```python
from build123d import *

# Parameters (mm, degrees)
F1_DEPTH = 127
F1_TAPER = -10
F2_R     = 7.8205252783
F3_DEPTH = 127.0010001
F4_R     = 16.8280941537
F5_DEPTH = 127.0010001
F6_W     = 92.6431566477
F6_H     = 12.3323691078
F7_DEPTH = 127.0010001


with BuildPart() as f1:
    # F0 (on Front) → F1 (new body)
    with BuildSketch(Plane.XZ):
        Polygon((-16.393026337, 9.7756581381), (-47.3743416369, 15.1898693293), (-52.7885518968, 0), (61.8122331798, 0), (61.8122331798, 17.2953940928), (29.9285557121, 10.07644739), (4.6622389928, 23.0103954673), align=None)
    extrude(amount=F1_DEPTH, taper=F1_TAPER)

    # F2 (on face) → F3 (cut, through all)
    with BuildSketch(Plane.XZ.offset(127)):
        with Locations((45.4005300999, 11.279605329)):
            Circle(F2_R)
    extrude(amount=-F3_DEPTH, mode=Mode.SUBTRACT)

    # F4 (on face) → F5 (cut, through all)
    with BuildSketch(Plane.XZ.offset(127)):
        with Locations((-42.574852705, 18.9597774297)):
            Circle(F4_R)
    extrude(amount=-F5_DEPTH, mode=Mode.SUBTRACT)

    # F6 (on face) → F7 (cut, through all)
    with BuildSketch(Plane.XZ.offset(127)):
        with Locations((3.5907924175, -9.3244740274)):
            Rectangle(F6_W, F6_H)
    extrude(amount=-F7_DEPTH, mode=Mode.SUBTRACT)


solid = f1.part
```
Geometry: final body of the model. Coordinates: model frame, mm. A direction names the side the tool comes from. Round coordinates to 2 decimals unless told otherwise and drop trailing zeros. Use CSV: the item, a comma, the result in double quotes. Start each with the question number.
Q1. Line query: L1, parallel to Z at x = -57, y = -107; L2, parallel to X at y = -97.5, z = 23; L3, parallel to X at y = -26.5, z = 12.5. Output: solid intervals per line, ascending.
Q2. First-contact query: pin 1 Ø2 at (y, z) = (-113.5, 30) entering from -X; pin 2 Ø12 at (x, y) = (-23.5, -107.5) entering from -Z; pin 3 Ø19.5 at (x, y) = (-3, -107) entering from +Z. Flat tips, straight axial feed; report the tip coordinate or a pass-through.
Q3. Pull-direction query (X, two-part tool) for faces 3 (the face through (8, -127, 6)), 4 (the face through (49.01, -64.39, 4.34)); classes: pulls with the +X half, pulls with the -X half, needs draft (parallel to the pull), parting line crosses it, or undercut.
Q4. Section A-A (y = -91.5). Give the number of separate pieces and of enclosed holes in the cut face, plus the area to 3 significant figures.
Q5. Reachability of faces 1 (the face through (9, 0, 7)), 2 (the face through (3, -73, -3.158)) from +Z, -Z, +X, -X, +Y, -Y: full face, straight path, thin tool, end or side. Return the list, or none.
Result sheet:
1,L1,"-18.87 to 10.29, 27.63 to 36.02"
1,L2,"-62.84 to -58.91, -26.24 to 79"
1,L3,"-27.04 to 37.68, 53.13 to 66.48"
2,pin 1,"x = -63.74"
2,pin 2,"z = -20.01"
2,pin 3,"z = 46.14"
3,face 3,"needs draft"
3,face 4,"undercut"
4,separate pieces,"1"
4,enclosed holes,"2"
4,area,"4,900 mm²"
5,face 1,"+Z, -Z, +X, -X, +Y"
5,face 2,"+Y, -Y"
